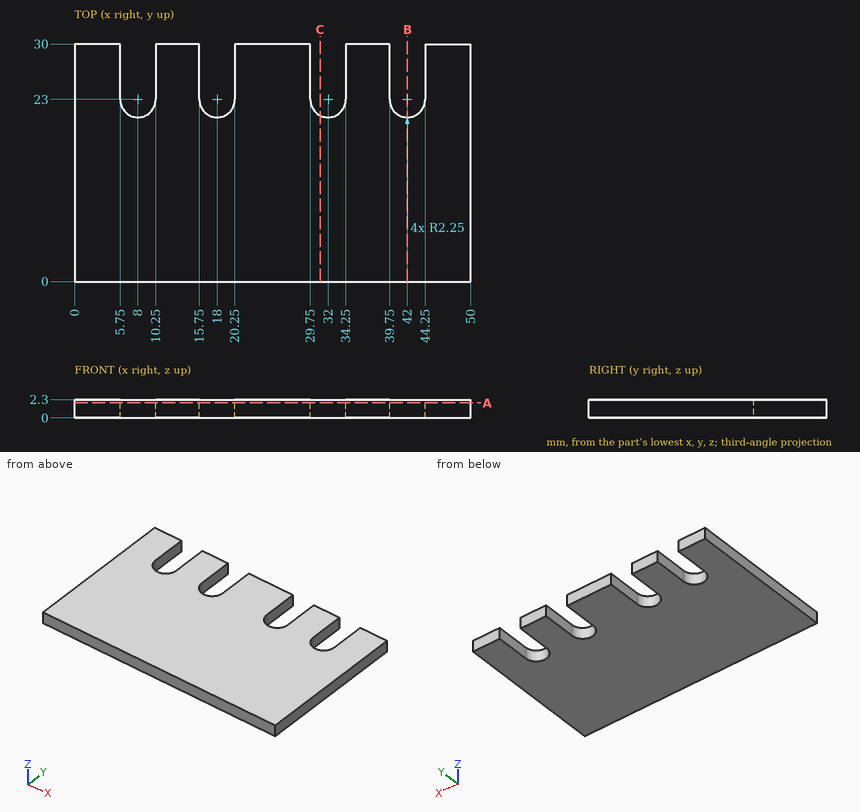
Can you work these out from the drawing? Everything is in mm from the part's minimum corner. Give positions to 0.01 mm unless a question says otherwise; leave off trailing zeros. Order: outer loops, then holes, each group sorted by start corner. A loop starts at its lowest first (then second) coordinate and runs counter-clockwise, first axis right, second up.
1. Suppose I cut it at A-A (z = 1.9). List the corners of the cut face in (x, y) for me.
2. I need wall thicknesses on L1, parallel to X at y = 25.25, z = 0.5; L2, parallel to X at y = 22.25, z = 1.1; L3, parallel to Y at x = 34, z = 1.6. Which ranges of each line are inside material? Lowest first, please.
3. Suppose I cut it at B-B (x = 42). List the corners of the cut face in (y, z) for me.
4. Suppose I cut it at C-C (x = 31). List the corners of the cut face in (y, z) for me, plus the area to 3 significant figures.
Solved:
1. outline: (0, 0) - (50, 0) - (50, 30) - (44.25, 30) - (44.25, 23) arc R2.25 cw to (39.75, 23) - (39.75, 30) - (34.25, 30) - (34.25, 23) arc R2.25 cw to (29.75, 23) - (29.75, 30) - (20.25, 30) - (20.25, 23) arc R2.25 cw to (15.75, 23) - (15.75, 30) - (10.25, 30) - (10.25, 23) arc R2.25 cw to (5.75, 23) - (5.75, 30) - (0, 30) - close
2. L1: x = 0 to 5.75, 10.25 to 15.75, 20.25 to 29.75, 34.25 to 39.75, 44.25 to 50
2. L2: x = 0 to 5.88, 10.12 to 15.88, 20.12 to 29.88, 34.12 to 39.88, 44.12 to 50
2. L3: y = 0 to 21.97
3. outline: (0, 0) - (20.75, 0) - (20.75, 2.3) - (0, 2.3) - close
4. outline: (0, 0) - (20.98, 0) - (20.98, 2.3) - (0, 2.3) - close
4. area: 48.3 mm2
